from build123d import *

# Parameters (mm, degrees)
F0_R     = 4.5
F1_DEPTH = 3
F0_R_2   = 3.5
F2_DEPTH = 5


with BuildPart() as f1:
    # F0 (on Top) → F1 (new body)
    with BuildSketch(Plane.XY):
        with BuildLine():
            ThreePointArc((0, 0), (-0.860465, 3.488061), (-3.244419, 6.175762))
            ThreePointArc((-3.244419, 6.175762), (-15, 0), (-3.244419, -6.175762))
            ThreePointArc((-3.244419, -6.175762), (-0.860465, -3.488061), (0, 0))
        make_face()
        with Locations((-7.5, 0)):
            Circle(F0_R, mode=Mode.SUBTRACT)
        with BuildLine():
            ThreePointArc((15, 0), (10.988061, 6.639535), (3.244419, 6.175762))
            ThreePointArc((3.244419, 6.175762), (0.860465, 3.488061), (0, 0))
            ThreePointArc((0, 0), (0.860465, -3.488061), (3.244419, -6.175762))
            ThreePointArc((3.244419, -6.175762), (10.988061, -6.639535), (15, 0))
        make_face()
        with Locations((7.5, 0)):
            Circle(F0_R, mode=Mode.SUBTRACT)
        with BuildLine():
            Line((3.244419, 6.175762), (-3.244419, 6.175762))
            ThreePointArc((-3.244419, 6.175762), (-0.860465, 3.488061), (0, 0))
            ThreePointArc((0, 0), (0.860465, 3.488061), (3.244419, 6.175762))
        make_face()
        with BuildLine():
            ThreePointArc((3.244419, -6.175762), (0.860465, -3.488061), (0, 0))
            ThreePointArc((0, 0), (-0.860465, -3.488061), (-3.244419, -6.175762))
            Line((-3.244419, -6.175762), (3.244419, -6.175762))
        make_face()
    extrude(amount=-F1_DEPTH)

    # F0 (on Top) → F2 (join)
    with BuildSketch(Plane.XY):
        with Locations((7.5, 0)):
            Circle(F0_R)
        with Locations((7.5, 0)):
            Circle(F0_R_2, mode=Mode.SUBTRACT)
        with Locations((-7.5, 0)):
            Circle(F0_R)
        with Locations((-7.5, 0)):
            Circle(F0_R_2, mode=Mode.SUBTRACT)
    extrude(amount=-F2_DEPTH)


solid = f1.part
Model file for the job. Use its own axes, mm. A direction names the side the tool comes from. Round coordinates to 2 decimals unless told otherwise and drop trailing zeros. Loops run counter-clockwise (first coordinate to the right, second up) from the corner with the lowest first, then second, coordinate; pieces in that order, holes last.
1. Drop flat-ended pins along their axis: P1, Ø1.5, axis at x = 1, z = -1.5, coming from the +Y side; P2, Ø1.5, axis at x = -0.5, z = -3, coming from the -Y side. Give the stop position or say it passes through.
Check values:
P1: stops at y = 6.18
P2: stops at y = -6.18
2. Tool access for faces 5 (the flat face through (0, 6.176, -1)), 6 (the cylindrical face through (-3.208, 1.352, -3.986)), 7 (the flat face through (-5, -3, -5)): list every direction of +Z, -Z, +X, -X, +Y, -Y with a clear straight run to the whole face (end or side of a thin tool).
Check values:
face 5: +Z, -Z, +Y
face 6: -Z
face 7: -Z, +X, -X, +Y, -Y
3. Band-saw the part on C-C, the plane z = -0.9. List the corners of the cut face in (x, y).
Check values:
outline: (-3.24, -6.18) - (3.24, -6.18) arc R7.5 ccw to (15, 0) arc R7.5 ccw to (3.24, 6.18) - (-3.24, 6.18) arc R7.5 ccw (long way) to start; hole circle Ø7 at (-7.5, 0); hole circle Ø7 at (7.5, 0)
4. Band-saw the part on D-D, the plane y = -3. List the corners of the cut face in (x, z).
Check values:
outline: (-14.37, -3) - (-10.85, -3) - (-10.85, -5) - (-9.3, -5) - (-9.3, 0) - (-14.37, 0) - close; (-5.7, -5) - (-4.15, -5) - (-4.15, -3) - (4.15, -3) - (4.15, -5) - (5.7, -5) - (5.7, 0) - (-5.7, 0) - close; (9.3, -5) - (10.85, -5) - (10.85, -3) - (14.37, -3) - (14.37, 0) - (9.3, 0) - close
5. Wall check: probe 1 along Y at (x, z) = (7.5, -1.15); probe 2 along X at (y, z) = (2.75, -4.1); probe 3 along X at (y, z) = (3, -2.2). Give the ranges that are in metal, low to high.
Check values:
probe 1: y = -7.5 to -3.5, 3.5 to 7.5
probe 2: x = -11.06 to -9.67, -5.33 to -3.94, 3.94 to 5.33, 9.67 to 11.06
probe 3: x = -14.37 to -9.3, -5.7 to 5.7, 9.3 to 14.37
6. Mould opens along Y. For faces 1 (the flat face through (0, -6.176, -1)), 2 (the cylindrical face through (-11, 0, -2)), 3 (the flat face through (0, 0, -3)), 4 (the cylindrical face through (11.792, 1.352, -3.986)) say: +Y half, -Y half, draft (parallel to the pull), parting line (faces both ways), or undercut.
Check values:
face 1: -Y half
face 2: undercut
face 3: draft
face 4: parting line
7. Band-saw the part on B-B, the plane y = 6.75. List the corners of the cut face in (x, z).
Check values:
outline: (-10.77, -3) - (-4.23, -3) - (-4.23, 0) - (-10.77, 0) - close; (4.23, -3) - (10.77, -3) - (10.77, 0) - (4.23, 0) - close
8. Band-saw the part on A-A, the plane x = -7.5. List the corners of the cut face in (y, z), and give its area (3 significant figures).
Check values:
outline: (-7.5, -3) - (-4.5, -3) - (-4.5, -5) - (-3.5, -5) - (-3.5, 0) - (-7.5, 0) - close; (3.5, -5) - (4.5, -5) - (4.5, -3) - (7.5, -3) - (7.5, 0) - (3.5, 0) - close
area: 28.0 mm2
